Geometry check sheet. Reference: the model listing, model coordinates, mm. Round coordinates to 2 decimals unless told otherwise and drop trailing zeros. Loops run counter-clockwise (first coordinate to the right, second up) from the corner with the lowest first, then second, coordinate; pieces in that order, holes last. Notation, with made-up numbers: (-26, 29.25) - (2, 29.25) arc R27 cw to (2, 68.25) - close; hole circle Ø3 at (-16.5, -1.5). An arc over 180 degrees is marked (long way). Answer as CSV lines item,"result". Start each with the question number.
1) Depth check by flat-ended pin: P1, Ø1, axis at y = -19.5, z = 0.5, coming from the -X side; P2, Ø5.5, axis at x = 0, y = 0, coming from the +Z side; P3, Ø1, axis at y = 3, z = 1.5, coming from the -X side. Enter the tip coordinate at first touch or a pass-through.
2) Cross-section at A-A on x = -4.5. Record the boundary of the cut face in (y, z).
3) Cross-section at B-B on y = -7. Record the boundary of the cut face in (x, z).
4) Thickness scan on line 1 along Y through (x, z) = (-9, 1.4); line 2 along Y through (x, z) = (14, 2.15); line 3 along Y through (x, z) = (23, 0.15). Record the ranges inside material, lowest first.
5) Cross-section at D-D on x = -12. Record the boundary of the cut face in (y, z).
6) Cross-section at C-C on z = 0.9. Record the boundary of the cut face in (x, y) (1 decimal).
from build123d import *

# Parameters (mm, degrees)
F0_R     = 2.465
F1_DEPTH = 2.38


with BuildPart() as f1:
    # F0 (on Top) → F1 (new body)
    with BuildSketch(Plane.XY):
        with BuildLine():
            ThreePointArc((0, 10), (4.359747, 8.999589), (7.847187, 6.198521))
            ThreePointArc((7.847187, 6.198521), (8.410225, 12.486219), (10.984446, 18.25038))
            ThreePointArc((10.984446, 18.25038), (13.553523, 19.219431), (16.124126, 18.254435))
            ThreePointArc((16.124126, 18.254435), (14.432203, 20.69641), (12.065989, 22.49276))
            ThreePointArc((12.065989, 22.49276), (-2.422788, 26.778203), (-16.925003, 22.538461))
            ThreePointArc((-16.925003, 22.538461), (-6.056439, 19.517047), (0, 10))
        make_face()
        with BuildLine():
            ThreePointArc((-8.660254, -5), (-9.973746, -0.724143), (-9.29167, 3.696602))
            ThreePointArc((-9.29167, 3.696602), (-15.018496, 1.040359), (-21.297516, 0.38762))
            ThreePointArc((-21.297516, 0.38762), (-23.421277, 2.12798), (-23.870867, 4.836685))
            ThreePointArc((-23.870867, 4.836685), (-25.139718, 2.15045), (-25.512296, -0.796927))
            ThreePointArc((-25.512296, -0.796927), (-21.97921, -15.487297), (-11.056378, -25.926713))
            ThreePointArc((-11.056378, -25.926713), (-13.874039, -15.003553), (-8.660254, -5))
        make_face()
        with BuildLine():
            ThreePointArc((27.981381, 3.388252), (19.930478, -4.513494), (8.660254, -5))
            ThreePointArc((8.660254, -5), (5.613999, -8.275446), (1.444483, -9.895123))
            ThreePointArc((1.444483, -9.895123), (6.60827, -13.526578), (10.313069, -18.638))
            ThreePointArc((10.313069, -18.638), (9.867754, -21.347411), (7.746741, -23.09112))
            ThreePointArc((7.746741, -23.09112), (10.707515, -22.84686), (13.446307, -21.695833))
            ThreePointArc((13.446307, -21.695833), (24.401998, -11.290906), (27.981381, 3.388252))
        make_face()
        with BuildLine():
            ThreePointArc((8.660254, -5), (9.659258, -2.58819), (10, 0))
            ThreePointArc((10, 0), (9.446477, 3.280864), (7.847187, 6.198521))
            ThreePointArc((7.847187, 6.198521), (4.359747, 8.999589), (0, 10))
            ThreePointArc((0, 10), (-5.613999, 8.275446), (-9.29167, 3.696602))
            ThreePointArc((-9.29167, 3.696602), (-9.973746, -0.724143), (-8.660254, -5))
            ThreePointArc((-8.660254, -5), (-4.359747, -8.999589), (1.444483, -9.895123))
            ThreePointArc((1.444483, -9.895123), (5.613999, -8.275446), (8.660254, -5))
        make_face()
        Circle(F0_R, mode=Mode.SUBTRACT)
    extrude(amount=F1_DEPTH)


solid = f1.part
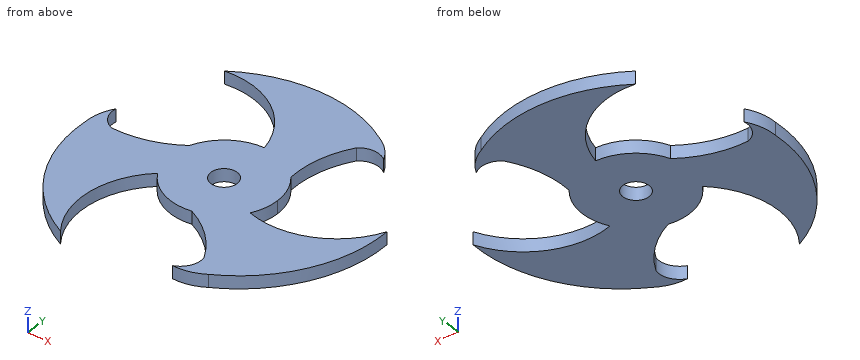
Answer block:
1,P1,"stops at x = -19.57"
1,P2,"stops at z = 2.38"
1,P3,"stops at x = -25.03"
2,outline,"(-8.93, 0) - (8.93, 0) - (8.93, 2.38) - (-8.93, 2.38) - close; (18.2, 0) - (26.7, 0) - (26.7, 2.38) - (18.2, 2.38) - close"
3,outline,"(-25.1, 0) - (-10.56, 0) - (-10.56, 2.38) - (-25.1, 2.38) - close; (-7.14, 0) - (26.4, 0) - (26.4, 2.38) - (-7.14, 2.38) - close"
4,line 1,"y = -5.31 to 4.36, 21.24 to 25.97"
4,line 2,"y = -21.4 to -5.81, 19.19 to 21.12"
4,line 3,"y = -13.46 to -2.75"
5,outline,"(-25.42, 0) - (-24.43, 0) - (-24.43, 2.38) - (-25.42, 2.38) - close; (-9.16, 0) - (2.15, 0) - (2.15, 2.38) - (-9.16, 2.38) - close; (22.23, 0) - (25.02, 0) - (25.02, 2.38) - (22.23, 2.38) - close"
6,outline,"(-25.5, -0.8) arc R26.8 ccw to (-11.1, -25.9) arc R15.7 cw to (-8.7, -5) arc R10 ccw to (1.4, -9.9) arc R19.2 cw to (10.3, -18.6) arc R3.9 cw to (7.7, -23.1) arc R9.5 ccw to (13.4, -21.7) arc R26.8 ccw to (28, 3.4) arc R15.7 cw to (8.7, -5) arc R10 ccw to (10, 0) arc R10 ccw to (7.8, 6.2) arc R19.2 cw to (11, 18.3) arc R3.9 cw to (16.1, 18.3) arc R9.5 ccw to (12.1, 22.5) arc R26.8 ccw to (-16.9, 22.5) arc R15.7 cw to (0, 10) arc R10 ccw to (-9.3, 3.7) arc R19.2 cw to (-21.3, 0.4) arc R3.9 cw to (-23.9, 4.8) arc R9.5 ccw to start; hole circle Ø4.9 at (0, 0)"
